Source: CAD feature listing. Evaluate the final solid. Frame: model axes, mm. Round coordinates to 2 decimals unless told otherwise and drop trailing zeros. Write each loop counter-clockwise with the first axis right and the second up, starting at its lowest first coordinate (ties: lowest second). Pieces come first, ordered by that corner, then holes. Notation, with made-up numbers: M 13.25,-25.75 L 45.25,-25.75 A12 ccw 45.25,-4.75 Z; hole C 44,49.25 d9. An arc over 180 degrees is marked long. Answer in a Markdown table with one row per item. Add a question column.
Item 1: Cut plane B-B on x = 10.5. Return loops of the section in (y, z).
Item 2: Material intervals for probe 1 along Y at (x, z) = (33.5, 16.75); probe 2 along Y at (x, z) = (45, 7.75); probe 3 along X at (y, z) = (13.5, 13.5), sorted ascending.
Item 3: Cut plane A-A on z = 20.25. Return loops of the section in (x, y), and give its area (3 significant figures).
Item 4: Contact query for flat-ended pins moving along their axis: pin 1 (6 mm diameter, centred on y = 9.5, z = 9.5, fed in from +X); pin 2 (8 mm diameter, centred on x = 49.5, z = 19, fed in from +Y); pin 3 (1 mm diameter, centred on x = 27.5, y = 4.5, fed in from -Z); pin 4 (8 mm diameter, centred on x = 37, y = 13, fed in from -Z). Output: stop coordinate, or through.
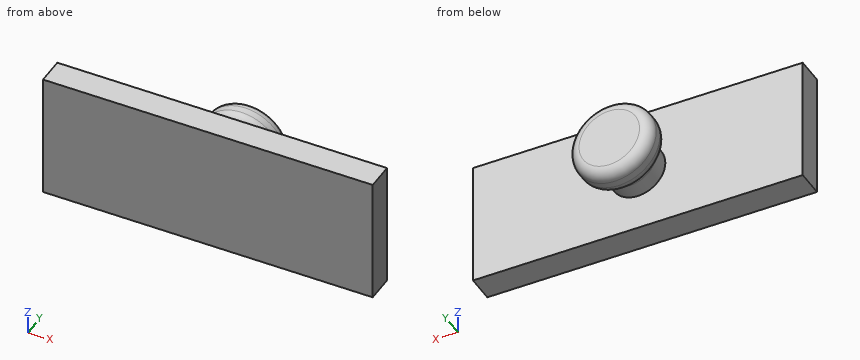
Autodesk Fusion 360 part; units mm, degrees
sketch "Sketch1" plane through (0, 0, 0) normal (0, 1, 0) x (1, 0, 0)
  line L0 (0, 0) -> (60, 0)
  line L1 (60, 0) -> (60, -23)
  line L2 (60, -23) -> (0, -23)
  line L3 (0, -23) -> (0, 0)
  dimension "d1" = 60
  dimension "d2" = 23
extrude "Extrude1" add sketch "Sketch1" along normal blind 5
sketch "Sketch2" plane through (0, 5, 0) normal (0, 1, 0) x (-1, 0, 0)
  line L0 (0, 23) -> (-60, 23)
  line L1 (-60, 23) -> (-60, 0)
  line L2 (-60, 0) -> (0, 0)
  line L3 (0, 0) -> (0, 23)
  circle A0 centre (-30, 11.5) radius 5
  dimension "d5" = 10
extrude "Extrude2" add sketch "Sketch2" along normal blind 5 contours A0
sketch "Sketch3" plane through (0, 10, 0) normal (0, 1, 0) x (-1, 0, 0)
  circle A0 centre (-30, 11.5) radius 5
  circle A1 centre (-30, 11.5) radius 7.5
  dimension "d8" = 15
extrude "Extrude3" add sketch "Sketch3" along normal blind 5 contours A0 | A1
fillet "Fillet1" radius 2 1 edges at (34.6616, 10, 9.6919)
fillet "Fillet2" radius 2 2 edges at (36.9925, 10, 8.7879) (36.9925, 15, 8.7879)
Results below:
| question | item | result |
|---|---|---|
| 1 | outline | M 0,0 L 5,0 L 5,23 L 0,23 Z |
| 2 | probe 1 | 0 to 5, 9.88 to 14.83 |
| 2 | probe 2 | 0 to 5 |
| 2 | probe 3 | 22.84 to 37.16 |
| 3 | outline | M 0,0 L 60,0 L 60,5 L 0,5 Z |
| 3 | area | 300 mm2 |
| 4 | pin 1 | x = 37.5 |
| 4 | pin 2 | y = 5 |
| 4 | pin 3 | z = 0 |
| 4 | pin 4 | z = 4.63 |
